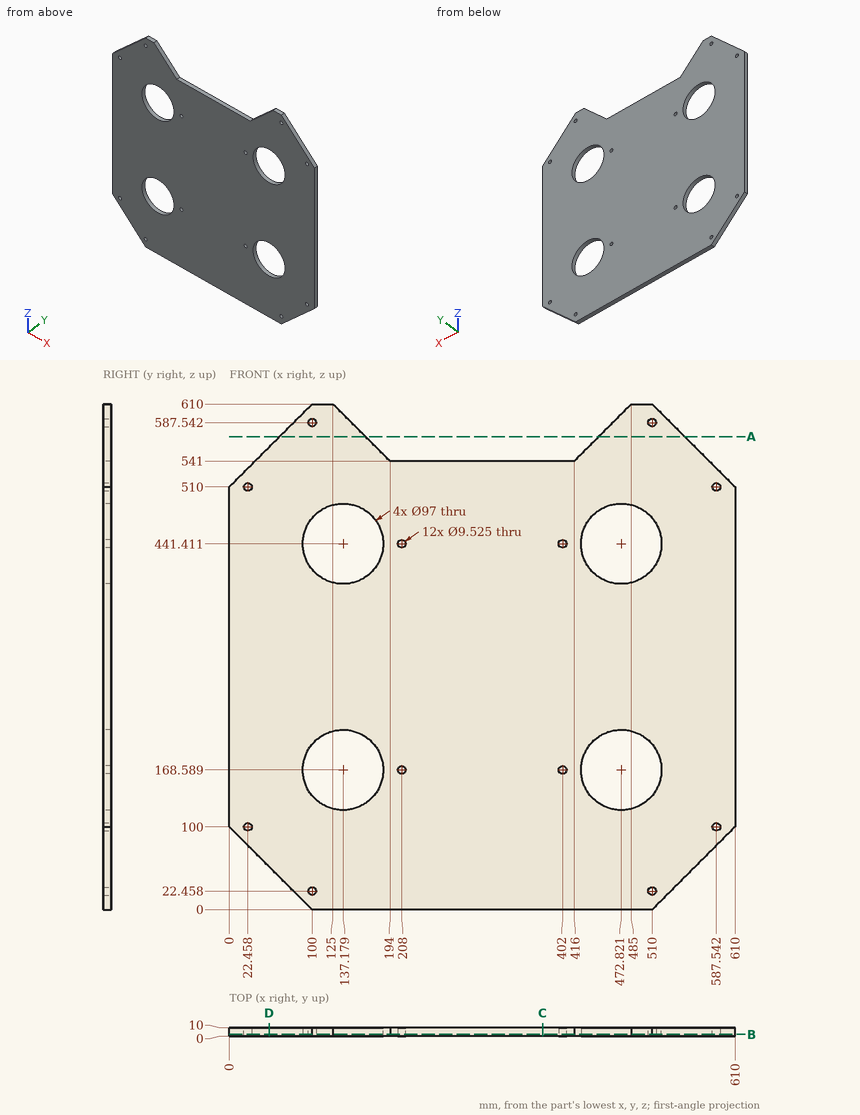
Source: three-view drawing plus pictorial views. Frame: mm from the lowest corner of the part. Coordinates: 2 decimals unless noted, no trailing zeros. Loops run counter-clockwise (first coordinate to the right, second up) from the corner with the lowest first, then second, coordinate; pieces in that order, holes last. Notation, with made-up numbers: (-18.75, 57.5) - (2.25, 57.5) arc R24 cw to (2.25, 69.5) - close; hole circle Ø5 at (-24.5, 58.25). An arc over 180 degrees is marked (long way). One line per item, written item: value. Start each with the question number.
1. Section B-B (y = 2). State how many separate pieces and enclosed holes the cut face has, and give its area (3 significant figures).
2. Section D-D (x = 48). Return the cut outline in (y, z).
3. Section C-C (x = 378). Return the cut outline in (y, z).
4. Ray query, L1, parallel to Z at x = 402, y = 5; L2, parallel to X at y = 4.5, z = 100 (1 decimal); L3, parallel to Z at x = 510, y = 2.75 (1 decimal). Return the intervals inside material, ascending.
5. Contact query for a flat-ended pin moving along its axis: P1, Ø4, axis at y = 4, z = 536, coming from the -X side. Output: stop coordinate, or through.
6. Section A-A (z = 570.5). Return the cut outline in (x, y), and give its area (3 significant figures).
Verdict:
1. separate pieces: 1
1. enclosed holes: 16
1. area: 302,000 mm2
2. outline: (0, 52) - (10, 52) - (10, 558) - (0, 558) - close
3. outline: (0, 0) - (10, 0) - (10, 541) - (0, 541) - close
4. L1: z = 0 to 163.83, 173.35 to 436.65, 446.17 to 541
4. L2: x = 0 to 17.7, 27.2 to 582.8, 592.3 to 610
4. L3: z = 0 to 17.7, 27.2 to 137.4, 199.7 to 410.3, 472.6 to 582.8, 592.3 to 610
5. P1: stops at x = 24
6. outline: (60.5, 0) - (164.5, 0) - (164.5, 10) - (60.5, 10) - close; (445.5, 0) - (549.5, 0) - (549.5, 10) - (445.5, 10) - close
6. area: 2,080 mm2
